```python
from build123d import *

# Parameters (mm, degrees)
SKETCH1_R           = 10.65
BOSS_EXTRUDE1_DEPTH = 1.6
SKETCH2_R           = 0.35
CUT_EXTRUDE1_DEPTH  = 44.909166683
SKETCH3_R           = 4
CUT_EXTRUDE2_DEPTH  = 44.909166683
SKETCH7_R           = 0.35
CUT_EXTRUDE6_DEPTH  = 10


with BuildPart() as part:
    # Sketch1 → Boss-Extrude1 (new body)
    with BuildSketch(Plane(origin=(0, 0, 0), x_dir=(1, 0, 0), z_dir=(0, 1, 0))):
        with Locations(Location((-21.736320014, 18.957113921, 0), (0, 0, 270))):
            Circle(SKETCH1_R)
    extrude(amount=BOSS_EXTRUDE1_DEPTH)

    # Sketch2 → Cut-Extrude1 (cut, through all)
    with BuildSketch(Plane(origin=(0, 1.6, 0), x_dir=(1, 0, 0), z_dir=(0, 1, 0))):
        with Locations(Location((-27.142133221, 21.560416356, 0), (0, 0, 270))):
            Circle(SKETCH2_R)
        with Locations(Location((-25.477258825, 23.648102816, 0), (0, 0, 270))):
            Circle(SKETCH2_R)
        with Locations(Location((-23.071445617, 24.806681394, 0), (0, 0, 270))):
            Circle(SKETCH2_R)
        with Locations(Location((-16.330506806, 21.560416356, 0), (0, 0, 270))):
            Circle(SKETCH2_R)
        with Locations(Location((-15.736320014, 18.957113921, 0), (0, 0, 270))):
            Circle(SKETCH2_R)
        with Locations(Location((-16.330506806, 16.353811486, 0), (0, 0, 270))):
            Circle(SKETCH2_R)
        with Locations(Location((-17.995381203, 14.266125026, 0), (0, 0, 270))):
            Circle(SKETCH2_R)
        with Locations(Location((-20.40119441, 13.107546448, 0), (0, 0, 270))):
            Circle(SKETCH2_R)
        with Locations(Location((-23.071445617, 13.107546448, 0), (0, 0, 270))):
            Circle(SKETCH2_R)
        with Locations(Location((-25.477258825, 14.266125026, 0), (0, 0, 270))):
            Circle(SKETCH2_R)
        with Locations(Location((-27.142133221, 16.353811486, 0), (0, 0, 270))):
            Circle(SKETCH2_R)
        with Locations(Location((-27.736320014, 18.957113921, 0), (0, 0, 270))):
            Circle(SKETCH2_R)
    extrude(amount=-CUT_EXTRUDE1_DEPTH, mode=Mode.SUBTRACT)

    # Sketch3 → Cut-Extrude2 (cut, through all)
    with BuildSketch(Plane(origin=(0, 1.6, 0), x_dir=(1, 0, 0), z_dir=(0, 1, 0))):
        with Locations(Location((-21.736320014, 18.957113921, 0), (0, 0, 270))):
            Circle(SKETCH3_R)
    extrude(amount=-CUT_EXTRUDE2_DEPTH, mode=Mode.SUBTRACT)

    # Sketch7 → Cut-Extrude6 (cut)
    with BuildSketch(Plane(origin=(0, 1.6, 0), x_dir=(1, 0, 0), z_dir=(0, 1, 0))):
        with Locations(Location((-27.760891742, 13.693604113, 0), (0, 0, 270))):
            Circle(SKETCH7_R)
        with Locations(Location((-29.448022899, 16.828819156, 0), (0, 0, 270))):
            Circle(SKETCH7_R)
        with Locations(Location((-29.607756722, 20.385569079, 0), (0, 0, 270))):
            Circle(SKETCH7_R)
        with Locations(Location((-28.208455969, 23.659395939, 0), (0, 0, 270))):
            Circle(SKETCH7_R)
        with Locations(Location((-25.527269313, 26.001878176, 0), (0, 0, 270))):
            Circle(SKETCH7_R)
        with Locations(Location((-15.711748286, 24.220623728, 0), (0, 0, 270))):
            Circle(SKETCH7_R)
        with Locations(Location((-14.024617128, 21.085408685, 0), (0, 0, 270))):
            Circle(SKETCH7_R)
        with Locations(Location((-24.880520267, 11.600891741, 0), (0, 0, 270))):
            Circle(SKETCH7_R)
        with Locations(Location((-13.864883305, 17.528658763, 0), (0, 0, 270))):
            Circle(SKETCH7_R)
        with Locations(Location((-15.264184059, 14.254831903, 0), (0, 0, 270))):
            Circle(SKETCH7_R)
        with Locations(Location((-17.945370714, 11.912349666, 0), (0, 0, 270))):
            Circle(SKETCH7_R)
        with Locations(Location((-21.377401371, 10.965169389, 0), (0, 0, 270))):
            Circle(SKETCH7_R)
    extrude(amount=-CUT_EXTRUDE6_DEPTH, mode=Mode.SUBTRACT)


solid = part.part
```
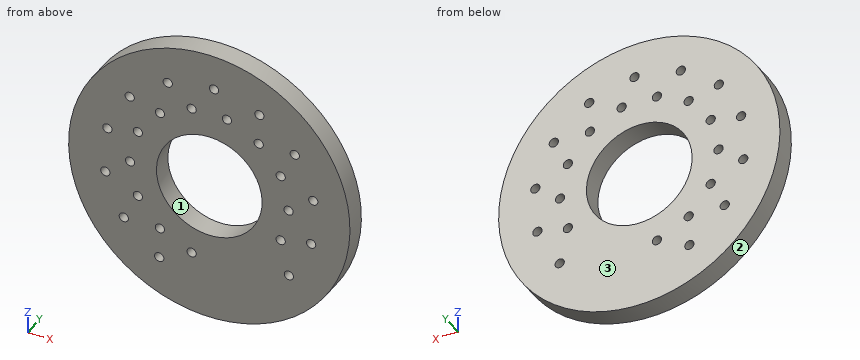
Can you work these out from the model? Positions are in its coordinate system, mm. Face numbers are marked on the shaded views. Coordinates: 2 decimals unless noted, no trailing zeros. Write each loop counter-clockwise with the first axis right and the second up, starting at its lowest first coordinate (ties: lowest second). Pieces come first, ordered by that corner, then holes. Notation, with made-up numbers: M 17.5,9 L 72.5,9 A27 cw 72.5,28 Z; hole C 47.5,-23.5 d10. An arc over 180 degrees is marked long. Answer as CSV lines item,"result".
Item 1: Please list where these lines run through material, in increasing order: line 1 along Z through (x, y) = (-23.25, 1.15); line 2 along X through (y, z) = (1.2, -19.25); line 3 along X through (y, z) = (0.7, -14).
Geometry results:
line 1,"z = -29.5 to -25.11, -24.51 to -22.66, -15.25 to -13.41, -12.81 to -8.42"
line 2,"x = -32.38 to -27.93, -27.54 to -25.73, -17.75 to -15.93, -15.54 to -11.09"
line 3,"x = -31.16 to -27.93, -27.59 to -25.7, -25.25 to -18.22, -17.77 to -15.5, -15.02 to -12.31"
Item 2: I'm going to push a flat-ended pin straight in: P1, Ø6.5, axis at x = -21.74, z = -18.96, coming from the -Y side. Where does the tip first touch, or does it pass through?
Geometry results:
P1,"passes through"
Item 3: Imagine slicing it at C-C on y = 0.85. State how many separate pieces and enclosed holes the cut face has, plus the area to 3 significant figures.
Geometry results:
separate pieces,"1"
enclosed holes,"25"
area,"297 mm2"
Item 4: Imagine slicing it at B-B on x = -24. List the corners of the cut face in (y, z) for me, plus the area to 3 significant figures.
Geometry results:
outline,"M 0,-29.36 L 1.6,-29.36 L 1.6,-22.25 L 0,-22.25 Z; M 0,-15.66 L 1.6,-15.66 L 1.6,-8.55 L 0,-8.55 Z"
area,"22.7 mm2"
Item 5: We'd pull the mould along Z, two halves only. Please class the marked faces 1, 2 and 3: +Z half, -Z half, draft (parallel to the pull), parting line (faces both ways), or undercut.
Geometry results:
face 1,"undercut"
face 2,"parting line"
face 3,"draft"
Item 6: Imagine slicing it at A-A on z = -15.5. List the corners of the cut face in (x, y) for me, plus the area to 3 significant figures.
Geometry results:
outline,"M -31.81,0 L -23.75,0 L -23.75,1.6 L -31.81,1.6 Z; M -19.72,0 L -11.66,0 L -11.66,1.6 L -19.72,1.6 Z"
area,"25.8 mm2"
Item 7: Imagine slicing it at D-D on z = -13. List the corners of the cut face in (x, y) for me, plus the area to 3 significant figures.
Geometry results:
outline,"M -30.56,0 L -23.4,0 L -23.4,1.6 L -30.56,1.6 Z; M -22.74,0 L -20.73,0 L -20.73,1.6 L -22.74,1.6 Z; M -20.07,0 L -12.91,0 L -12.91,1.6 L -20.07,1.6 Z"
area,"26.1 mm2"
